from build123d import *

# Parameters (mm, degrees)
SKETCH1_W             = 400.05
SKETCH1_H             = 127
BOSS_EXTRUDE1_DEPTH   = 6.35
SKETCH2_R             = 3.3655
CUT_EXTRUDE1_DEPTH    = 7.35
F_4_40_TAPPED_HOLE1_D = 2.2606


with BuildPart() as part:
    # Sketch1 → Boss-Extrude1 (new body)
    with BuildSketch(Plane.XY):
        Rectangle(SKETCH1_W, SKETCH1_H)
    extrude(amount=BOSS_EXTRUDE1_DEPTH)

    # Sketch2 → Cut-Extrude1 (cut, through all)
    with BuildSketch(Plane(origin=(0, 0, 0), x_dir=(-1, 0, 0), z_dir=(0, 0, -1))):
        with Locations((-180.975, -50.8)):
            Circle(SKETCH2_R)
        with Locations((-180.975, -25.4)):
            Circle(SKETCH2_R)
        with Locations((187.325, -50.8)):
            Circle(SKETCH2_R)
        with Locations((187.325, -25.4)):
            Circle(SKETCH2_R)
    extrude(amount=-CUT_EXTRUDE1_DEPTH, mode=Mode.SUBTRACT)

    # #4-40 Tapped Hole1 (through all)
    with Locations(Plane.XY.offset(6.35)):
        with Locations((-136.525, 45.025), (-136.525, 8.025), (-53.975, 45.025), (-53.975, 8.025), (28.575, 45.025), (28.575, 8.025), (111.125, 45.025), (111.125, 8.025)):
            Hole(F_4_40_TAPPED_HOLE1_D / 2)


solid = part.part
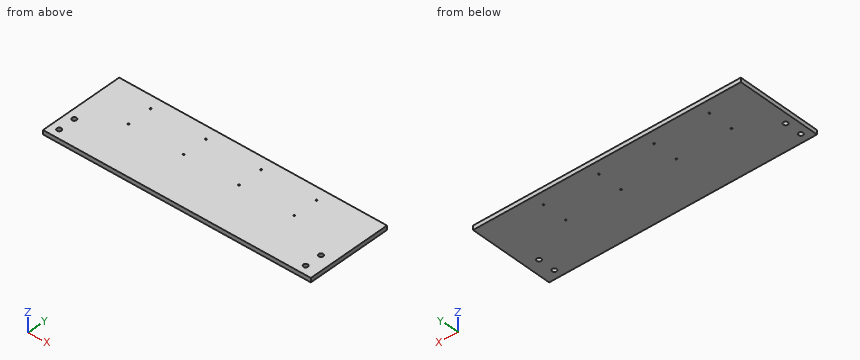
Build history of the part. All positions in model axes, mm. Round coordinates to 2 decimals unless told otherwise and drop trailing zeros. Write item = value, one per line.
(1) Band-saw the part on A-A (y = -25.4). State how many separate pieces and enclosed holes the cut face has, then the cut area to 3 significant figures.
Answer:
separate_pieces = 3
enclosed_holes = 0
area = 2,450 mm2
(2) Flat gauge pin, fed straight in: pin 1 (1.8 mm diameter, centred on x = -136.525, y = 45.025, fed in from +Z). Where does the tip first touch, or does it go through?
Answer:
pin_1 = through
(3) Probe L1, parallel to X at y = -28.5, z = 4 (3 decimals). List the from-to ranges inside material, lowest first.
Answer:
L1 = -200.025 to -188.635, -186.015 to 179.665, 182.285 to 200.025
